Autodesk Inventor part; units mm, degrees
ref_plane "YZ Plane" through (0, 0, 0) normal (1, 0, 0) x (0, 1, 0)
ref_plane "XZ Plane" through (0, 0, 0) normal (0, 1, 0) x (-1, 0, 0)
ref_plane "XY Plane" through (0, 0, 0) normal (0, 0, 1) x (1, 0, 0)
sketch "Sketch1" plane through (0, 0, 0) normal (0, 0, 1) x (1, 0, 0)
  line L0 (0, 0) -> (34, 0)
  line L1 (34, 0) -> (34, 40)
  line L2 (34, 40) -> (0, 40)
  line L3 (0, 40) -> (0, 0)
  line L4 (-6, 30) -> (0, 30)
  line L5 (0, 30) -> (0, 0)
  line L6 (0, 0) -> (-6, 0)
  line L7 (-6, 0) -> (-6, 30)
  line L8 (-6, 30) -> (0, 0) construction
  line L9 (0, 30) -> (-6, 0) construction
  line L10 (40, 30) -> (34, 30)
  line L11 (34, 30) -> (34, 0)
  line L12 (34, 0) -> (40, 0)
  line L13 (40, 0) -> (40, 30)
  line L14 (40, 30) -> (34, 0) construction
  line L15 (34, 30) -> (40, 0) construction
  line L16 (9.5, 32.5) -> (24.5, 32.5)
  line L17 (24.5, 32.5) -> (24.5, 7.5)
  line L18 (24.5, 7.5) -> (9.5, 7.5)
  line L19 (9.5, 7.5) -> (9.5, 32.5)
  line L20 (9.5, 32.5) -> (24.5, 7.5) construction
  line L21 (24.5, 32.5) -> (9.5, 7.5) construction
  point P0 (-3, 15)
  point P1 (37, 15)
  point P2 (0, 20)
  point P3 (0, 15)
  point P4 (34, 30)
  point P5 (0, 30)
  point P6 (17, 20)
  point P7 (17, 40)
  point P8 (34, 20)
  dimension "d0" = 34
  dimension "d1" = 40
  dimension "d2" = 6
  dimension "d3" = 6
  dimension "d4" = 30
  dimension "d5" = 30
  dimension "d8" = 15
  dimension "d9" = 25
extrude "Extrusion1" add sketch "Sketch1" along normal blind 3
properties part number "Frontrail"
Check sheet for the modelled part. Datum: model origin and axes. Units: mm. A direction names the side the tool comes from. Round coordinates to 2 decimals unless told otherwise and drop trailing zeros. Loops run counter-clockwise (first coordinate to the right, second up) from the corner with the lowest first, then second, coordinate; pieces in that order, holes last. Notation, with made-up numbers: (40.25, -39.75) - (65.25, -39.75) arc R21 cw to (65.25, -35.75) - close; hole circle Ø9 at (60, 60). An arc over 180 degrees is marked (long way). Answer as CSV lines item,"result". Start each with the question number.
Item 1: Section check B-B (y = 15). Record the boundary of the cut face in (x, z).
Item 2: Depth check by flat-ended pin: P1, Ø1.5, axis at y = 33, z = 1, coming from the +X side; P2, Ø1.5, axis at x = 36, z = 2, coming from the +Y side. Enter the tip coordinate at first touch or a pass-through.
Item 3: Section check A-A (z = 1.2). Record the boundary of the cut face in (x, y), and give its area (4 significant figures).
Item 4: Section check C-C (x = 21). Record the boundary of the cut face in (y, z), and give its area (3 significant figures).
Item 5: Release check for a two-part mould opening along X. For faces 5 (the flat face through (17, 7.5, 1)), 6 (the flat face through (40, 15, 1)), 7 (the flat face through (27, 20, 3)) record: +X half, -X half, draft (parallel to the pull), parting line (faces both ways), or undercut.
Item 6: Section check D-D (x = 35.5). Record the boundary of the cut face in (y, z).
Item 7: Scan lines: line 1 (X direction, y = 24.5, z = 1); line 2 (Y direction, x = 18, z = 1.55); line 3 (X direction, y = 37, z = 2.45). Record each from-to range of solid material in increasing order. Write a range as [from, to].
Item 8: Set-up check for faces 1 (the flat face through (17, 32.5, 1)), 2 (the flat face through (34, 35, 1)), 3 (the flat face through (-3, 30, 1)), 4 (the flat face through (27, 20, 0)): record each of +Z, -Z, +X, -X, +Y, -Y from which the full face is reachable in a straight line by a thin tool's end or side.
Report:
1,outline,"(-6, 0) - (9.5, 0) - (9.5, 3) - (-6, 3) - close; (24.5, 0) - (40, 0) - (40, 3) - (24.5, 3) - close"
2,P1,"stops at x = 34"
2,P2,"stops at y = 30"
3,outline,"(-6, 0) - (40, 0) - (40, 30) - (34, 30) - (34, 40) - (0, 40) - (0, 30) - (-6, 30) - close; hole (9.5, 7.5) - (24.5, 7.5) - (24.5, 32.5) - (9.5, 32.5) - close"
3,area,"1,345 mm2"
4,outline,"(0, 0) - (7.5, 0) - (7.5, 3) - (0, 3) - close; (32.5, 0) - (40, 0) - (40, 3) - (32.5, 3) - close"
4,area,"45.0 mm2"
5,face 5,"undercut"
5,face 6,"+X half"
5,face 7,"draft"
6,outline,"(0, 0) - (30, 0) - (30, 3) - (0, 3) - close"
7,line 1,"x = [-6, 9.5], [24.5, 40]"
7,line 2,"y = [0, 7.5], [32.5, 40]"
7,line 3,"x = [0, 34]"
8,face 1,"+Z, -Z"
8,face 2,"+Z, -Z, +X, +Y"
8,face 3,"+Z, -Z, -X, +Y"
8,face 4,"-Z, +X, -X, +Y, -Y"
